The model under review builds one solid part; all positions refer to its coordinate system, in mm. Coordinates: 2 decimals unless noted, no trailing zeros. Order: outer loops, then holes, each group sorted by start corner. A loop starts at its lowest first (then second) coordinate and runs counter-clockwise, first axis right, second up. Notation, with made-up numbers: (2.5, -29.5) - (35.5, -29.5) arc R29 ccw to (35.5, 8.5) - close; hole circle Ø2 at (22, -31.5). An arc over 180 degrees is marked (long way). Answer in a Markdown table with one row per item.
Autodesk Inventor part; units mm, degrees
ref_plane "YZ Plane" through (0, 0, 0) normal (1, 0, 0) x (0, 1, 0)
ref_plane "XZ Plane" through (0, 0, 0) normal (0, 1, 0) x (-1, 0, 0)
ref_plane "XY Plane" through (0, 0, 0) normal (0, 0, 1) x (1, 0, 0)
sketch "Sketch1" plane through (0, 0, 0) normal (0, 1, 0) x (-1, 0, 0)
  line L0 (93, -25) -> (-93, -25)
  line L1 (-93, -25) -> (-93, 25)
  line L2 (-93, 25) -> (93, 25)
  line L3 (93, 25) -> (93, -25)
  line L4 (93, -25) -> (-93, 25) construction
  line L5 (-93, -25) -> (93, 25) construction
  line L6 (17, 2) -> (-83, 2)
  line L7 (-83, 2) -> (-83, 17)
  line L8 (-83, 17) -> (17, 17)
  line L9 (17, 17) -> (17, 2)
  point P0 (0, 0)
  point P1 (-83, 9.5)
  point P2 (-33, 17)
  dimension "d0" = 186
  dimension "d1" = 50
  dimension "d20" = 10
  dimension "d21" = 100
  dimension "d23" = 23
  dimension "d24" = 8
extrude "Extrusion1" add sketch "Sketch1" along normal blind 3
chamfer "Chamfer3" distance 3 angle 45 1 edges at (-93, 0, 0) measured on face at (-93, 1, -8.3333)
chamfer "Chamfer4" distance 3 angle 45 1 edges at (93, 0, 0) measured on face at (93, 1, 8.3333)
properties part number "Back Wall"
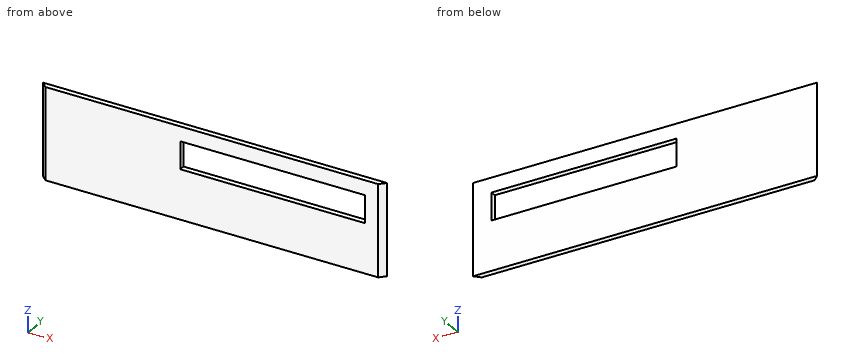
Item 1: To check wall thickness, follow line 1 (Z direction, x = 41, y = 0.65); line 2 (X direction, y = 0.85, z = 10.5); line 3 (X direction, y = 1.8, z = 19.5). State the ranges of each line that lie inside material, in increasing order. Write a range as from..to.
Check values:
| item | result |
|---|---|
| line 1 | -25..2, 17..25 |
| line 2 | -90.85..-17, 83..90.85 |
| line 3 | -91.8..91.8 |
Item 2: We need section C-C, the plane y = 1.25. Write out the cut boundary in (x, z).
Check values:
| item | result |
|---|---|
| outline | (-91.25, -25) - (91.25, -25) - (91.25, 25) - (-91.25, 25) - close; hole (-17, 2) - (83, 2) - (83, 17) - (-17, 17) - close |
Item 3: Clearance check with flat-ended pins moving along their axes: pin 1 Ø0.9 at (y, z) = (2, 12.5) entering from +X; pin 2 Ø1 at (y, z) = (1.5, 1.5) entering from -X; pin 3 Ø2 at (x, z) = (45, 14.5) entering from -Y. State where each tip first meets the part, or that it passes through.
Check values:
| item | result |
|---|---|
| pin 1 | x = 92.45 |
| pin 2 | x = -92 |
| pin 3 | through |
Item 4: We need section B-B, the plane x = 69. Write out the cut boundary in (y, z).
Check values:
| item | result |
|---|---|
| outline | (0, -25) - (3, -25) - (3, 2) - (0, 2) - close; (0, 17) - (3, 17) - (3, 25) - (0, 25) - close |
